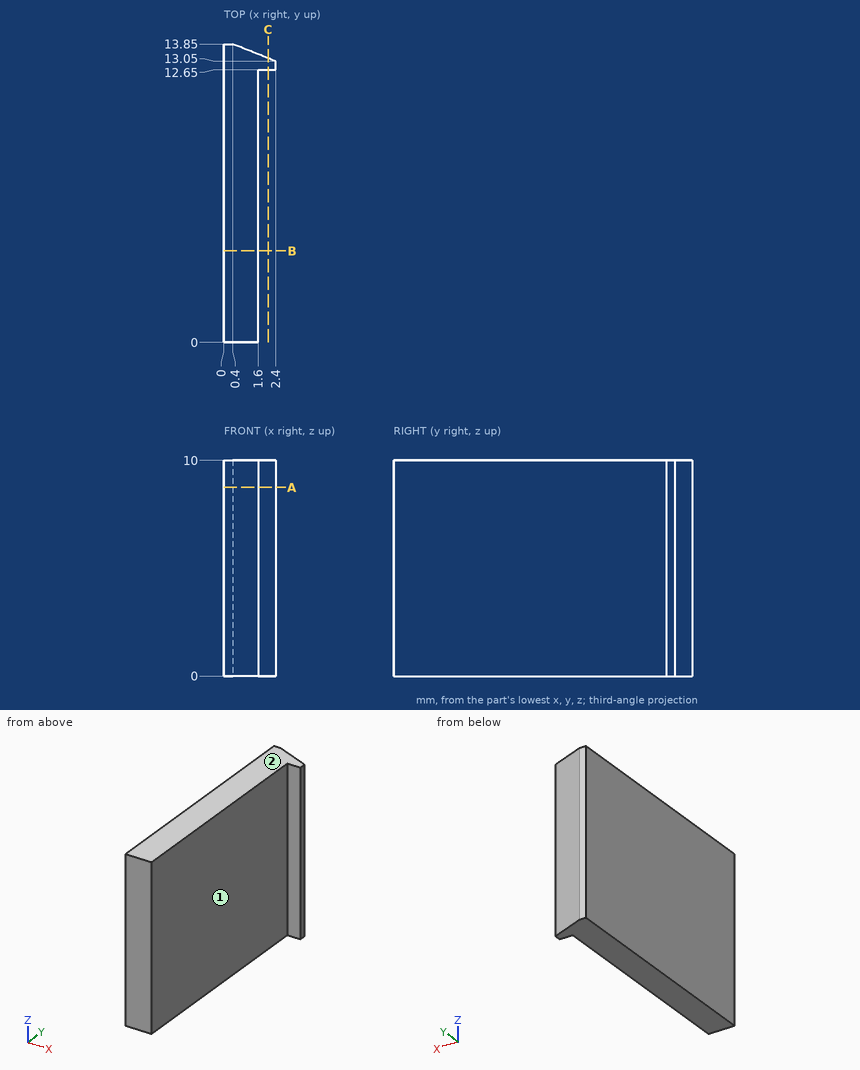
Drawing for the job (mm, zero at the part's lowest x, y, z). A direction names the side the tool comes from. Give positions to 0.01 mm unless a question says otherwise; leave off trailing zeros. Write each loop counter-clockwise with the first axis right and the second up, starting at its lowest first coordinate (ties: lowest second). Pieces come first, ordered by that corner, then holes. Notation, with made-up numbers: M 11.25,30 L 42.25,30 A28 ccw 42.25,48 Z; hole C 83.25,62 d4. An arc over 180 degrees is marked long. Use CSV: the item, a comma, the result in double quotes.
Item 1: Slice it at B-B on y = 4.25. Write the cut outline in (x, z).
Taken from the geometry:
outline,"M 0,0 L 1.6,0 L 1.6,10 L 0,10 Z"
Item 2: Which spindle directions (+Z, -Z, +X, -X, +Y, -Y) get a long thin tool onto all of the face, cutting with end or side? Do the marked faces 1 and 2. Say none if no direction does.
Taken from the geometry:
face 1,"+Z, -Z, +X, -Y"
face 2,"+Z, +X, -X, +Y, -Y"
Item 3: Slice it at C-C on x = 2.05. Write the cut outline in (y, z).
Taken from the geometry:
outline,"M 12.65,0 L 13.19,0 L 13.19,10 L 12.65,10 Z"
Item 4: Slice it at A-A on z = 8.75. Write the cut outline in (x, y), plus the area to 3 significant figures.
Taken from the geometry:
outline,"M 0,0 L 1.6,0 L 1.6,12.65 L 2.4,12.65 L 2.4,13.05 L 0.4,13.85 L 0,13.85 Z"
area,"22.3 mm²"
Item 5: Pin check, flat tips, straight feed: P1, Ø1, axis at x = 1, z = 7.5, coming from the +Y side; P2, Ø5, axis at y = 9, z = 7, coming from the +X side. Stop position of each tip, or through.
Taken from the geometry:
P1,"stops at y = 13.81"
P2,"stops at x = 1.6"
Item 6: Drill centre lines: probe 1 along X at (y, z) = (7.75, 7.5); probe 2 along Y at (x, z) = (2.2, 9); probe 3 along Y at (x, z) = (0.55, 6.25). Where is each one in solid material? Low to high.
Taken from the geometry:
probe 1,"x = 0 to 1.6"
probe 2,"y = 12.65 to 13.13"
probe 3,"y = 0 to 13.79"
